from build123d import *

# Parameters (mm, degrees)
BOSS_EXTRUDE1_DEPTH     = 70
SKETCH4_W               = 5
SKETCH4_H               = 20
BOSS_EXTRUDE2_DEPTH     = 20
CUT_EXTRUDE2_DEPTH      = 114.967153248
CUT_EXTRUDE2_DEPTH_BACK = 114.967153248
CUT_EXTRUDE3_REACH      = 115.967
SKETCH6_R               = 2.25
SKETCH7_R               = 3.75
CUT_EXTRUDE4_DEPTH      = 3
FILLET1_R               = 5


with BuildPart() as part:
    # Sketch1 → Boss-Extrude1 (new body)
    with BuildSketch(Plane.YZ):
        Polygon((-1.638304089, 85), (1.638304089, 87.294305745), (1.638304089, -87.294305745), (-1.638304089, -85), align=None)
    extrude(amount=BOSS_EXTRUDE1_DEPTH)

    # Sketch4 → Boss-Extrude2 (add)
    with BuildSketch(Plane(origin=(0, 1.638304089, 0), x_dir=(-1, 0, 0), z_dir=(0, 1, 0))):
        with Locations((-2.5, 0)):
            Rectangle(SKETCH4_W, SKETCH4_H)
    extrude(amount=BOSS_EXTRUDE2_DEPTH)

    # Sketch5 → Cut-Extrude2 (cut, two sides: drawn at the far end of the back side and taken through both)
    with BuildSketch(Plane(origin=(0, 0, 0), x_dir=(0, 1, 0), z_dir=(0, 0, 1)).offset(-CUT_EXTRUDE2_DEPTH_BACK)):
        with BuildLine():
            ThreePointArc((3.361695911, 0), (-0.173837995, -1.464466094), (-1.638304089, -5))
            Line((-1.638304089, -5), (-1.638304089, 0))
            Line((-1.638304089, 0), (3.361695911, 0))
        make_face()
    extrude(amount=CUT_EXTRUDE2_DEPTH + CUT_EXTRUDE2_DEPTH_BACK, mode=Mode.SUBTRACT)

    # Sketch6 → Cut-Extrude3 (cut, up to next)
    with BuildSketch(Plane(origin=(0, 0, 0), x_dir=(0, -1, 0), z_dir=(-1, 0, 0)), mode=Mode.PRIVATE) as cut_extrude3_sk1:
        with Locations(Location((-12.5, 0, 0), (0, 0, 90))):
            Circle(SKETCH6_R)
    cut_extrude3_tool1 = extrude(cut_extrude3_sk1.sketch, amount=-CUT_EXTRUDE3_REACH, mode=Mode.PRIVATE) & part.part
    add(cut_extrude3_tool1.solids().sort_by_distance((0, 12.5, 0))[0], mode=Mode.SUBTRACT)

    # Sketch7 → Cut-Extrude4 (cut)
    with BuildSketch(Plane(origin=(0, 0, 0), x_dir=(0, -1, 0), z_dir=(-1, 0, 0))):
        with Locations(Location((-12.5, 0, 0), (0, 0, 90))):
            Circle(SKETCH7_R)
    extrude(amount=-CUT_EXTRUDE4_DEPTH, mode=Mode.SUBTRACT)

    # Fillet1
    fillet1_edges = [part.edges().sort_by_distance(p)[0] for p in [
        (2.5, 21.638304089, -10),
        (2.5, 21.638304089, 10),
    ]]
    fillet(fillet1_edges, radius=FILLET1_R)


solid = part.part
Source: CAD feature listing. Evaluate the final solid. Frame: model axes, mm. A direction names the side the tool comes from. Coordinates: 2 decimals unless noted, no trailing zeros. Loops run counter-clockwise (first coordinate to the right, second up) from the corner with the lowest first, then second, coordinate; pieces in that order, holes last. Notation, with made-up numbers: (85, 29) - (127, 29) arc R19 ccw to (127, 48) - close; hole circle Ø8 at (-6.75, 75.25). An arc over 180 degrees is marked (long way). One line per item, written item: value. Start each with the question number.
1. Section A-A (z = 0). Return the cut outline in (x, y).
2. Set-up query: faces 1 (the flat face through (3, 9, -10)), 2 (the cylindrical face through (1.479, 16.218, -0.488)), 3 (the flat face through (3, 9, 10)), 4 (the cylindrical face through (2.087, -0.702, -1.222)), 5 (the flat face through (5, 9, 0)). Return all of +Z, -Z, +X, -X, +Y, -Y with unobstructed straight access to the full face (end or side cutting, diameter ignored); none if empty.
3. Mould query, pull axis Y, two halves, no side actions, for faces 6 (the flat face through (3, 11, 2)), 7 (the flat face through (34.67, 0.02, -86.16)), 8 (the cylindrical face through (3.99, 14.73, -0.29)), 9 (the flat face through (70, 0, 1)). Classes: pulls with the +Y half, pulls with the -Y half, needs draft (parallel to the pull), parting line crosses it, or undercut.
4. Section B-B (y = 12.5). Return the cut outline in (x, z), and give its area (3 significant figures).
5. Contact query for flat-ended pins moving along their axis: P1, Ø2.5, axis at x = 2.5, y = 8, coming from the -Z side; P2, Ø6, axis at y = 10.5, z = -0.5, coming from the -X side; P3, Ø7, axis at y = 12.5, z = 0, coming from the -X side; P4, Ø1.5, axis at x = 39.5, y = 1, coming from the -Z side. Output: stop coordinate, or through.
6. Section C-C (x = 40.5). Return the cut outline in (y, z), and give its area (3 significant figures).
7. Ray query, L1, parallel to Y at x = 63, z = -24; L2, parallel to Y at x = 1.8, z = 0; L3, parallel to Y at x = 1.1, z = 0. Return the intervals inside material, ascending.
8. Section D-D (z = -28). Return the cut outline in (x, y), and give its area (3 significant figures).
Verdict:
1. outline: (0, 3.36) arc R5 ccw to (5, -1.64) - (70, -1.64) - (70, 1.64) - (5, 1.64) - (5, 10.25) - (3, 10.25) - (3, 8.75) - (0, 8.75) - close; (0, 16.25) - (3, 16.25) - (3, 14.75) - (5, 14.75) - (5, 21.64) - (0, 21.64) - close
2. face 1: -Z, +X, -X, +Y
2. face 2: -X
2. face 3: +Z, +X, -X, +Y
2. face 4: +Z, -Z, -X, -Y
2. face 5: +Z, -Z, +X, +Y
3. face 6: undercut
3. face 7: pulls with the -Y half
3. face 8: undercut
3. face 9: needs draft
4. outline: (0, -10) - (5, -10) - (5, -2.25) - (3, -2.25) - (3, -3.75) - (0, -3.75) - close; (0, 3.75) - (3, 3.75) - (3, 2.25) - (5, 2.25) - (5, 10) - (0, 10) - close
4. area: 68.5 mm2
5. P1: stops at z = -10
5. P2: stops at x = 0
5. P3: stops at x = 3
5. P4: stops at z = -87.29
6. outline: (-1.64, -85) - (1.64, -87.29) - (1.64, 87.29) - (-1.64, 85) - close
6. area: 565 mm2
7. L1: y = -1.64 to 1.64
7. L2: y = -0.48 to 8.75, 16.25 to 21.64
7. L3: y = 0.23 to 8.75, 16.25 to 21.64
8. outline: (0.31, 1.64) arc R5 ccw to (5, -1.64) - (70, -1.64) - (70, 1.64) - close
8. area: 224 mm2
